Source: CAD feature listing. Evaluate the final solid. Frame: model axes, mm. Face numbers are marked on the shaded views. A direction names the side the tool comes from. Coordinates: 2 decimals unless noted, no trailing zeros. Write each loop counter-clockwise with the first axis right and the second up, starting at its lowest first coordinate (ties: lowest second). Pieces come first, ordered by that corner, then holes. Notation, with made-up numbers: (-23, -4.75) - (-19, -4.75) arc R33 ccw to (-19, 31.25) - close; hole circle Ø1 at (40, 56.5). An arc over 180 degrees is marked (long way). One line per question, with ' | ' between items.
from build123d import *

# Parameters (mm, degrees)
SKETCH1_R               = 17.5
BOSS_EXTRUDE1_DEPTH     = 4
BOSS_EXTRUDE2_DEPTH     = 6
CUT_EXTRUDE1_DEPTH      = 26.465663156
CUT_EXTRUDE1_DEPTH_BACK = 26.465663156
SKETCH3_R               = 1.6
CUT_EXTRUDE2_DEPTH      = 1
CUT_EXTRUDE2_DEPTH_BACK = 23.716032156
CUT_EXTRUDE2_START      = -2.749631
SKETCH5_R               = 2.1
CHAMFER1_SIZE           = 0.5
SKETCH6_R               = 3
CUT_EXTRUDE3_DEPTH      = 2


with BuildPart() as part:
    # Sketch1 → Boss-Extrude1 (new body)
    with BuildSketch(Plane(origin=(0, 0, 0), x_dir=(1, 0, 0), z_dir=(0, 1, 0))):
        with Locations(Location((0, 0, 0), (0, 0, 270))):
            Circle(SKETCH1_R)
    extrude(amount=BOSS_EXTRUDE1_DEPTH)

    # Sketch2 → Boss-Extrude2 (add)
    with BuildSketch(Plane(origin=(0, 0, 0), x_dir=(1, 0, 0), z_dir=(0, 1, 0))):
        with BuildLine():
            Line((-2.87, 6.929148577), (2.87, 6.929148577))
            ThreePointArc((2.87, 6.929148577), (0, -7.5), (-2.87, 6.929148577))
        make_face()
    extrude(amount=-BOSS_EXTRUDE2_DEPTH)

    # Sketch3 → Cut-Extrude1 (cut, two sides: drawn at the far end of the back side and taken through both)
    with BuildSketch(Plane(origin=(0, 0, 0), x_dir=(1, 0, 0), z_dir=(0, 1, 0)).offset(-CUT_EXTRUDE1_DEPTH_BACK)):
        with Locations(Location((0, 12.5, 0), (0, 0, 270))):
            Circle(SKETCH3_R)
        with Locations(Location((12.5, 0, 0), (0, 0, 270))):
            Circle(SKETCH3_R)
        with Locations(Location((0, -12.5, 0), (0, 0, 270))):
            Circle(SKETCH3_R)
        with Locations(Location((-12.5, 0, 0), (0, 0, 270))):
            Circle(SKETCH3_R)
        with BuildLine():
            Line((-1.5875, 2.749630657), (1.5875, 2.749630657))
            ThreePointArc((1.5875, 2.749630657), (0, -3.175), (-1.5875, 2.749630657))
        make_face()
    extrude(amount=CUT_EXTRUDE1_DEPTH + CUT_EXTRUDE1_DEPTH_BACK, mode=Mode.SUBTRACT)

    # Sketch5 → Cut-Extrude2 (cut, two sides: drawn at the far end of the back side and taken through both)
    with BuildSketch(Plane.XY.offset(CUT_EXTRUDE2_START - CUT_EXTRUDE2_DEPTH_BACK)):
        with Locations(Location((0, -3, 0), (0, 0, 180))):
            Circle(SKETCH5_R)
    extrude(amount=CUT_EXTRUDE2_DEPTH + CUT_EXTRUDE2_DEPTH_BACK, mode=Mode.SUBTRACT)

    # Chamfer1
    chamfer1_edges = [part.edges().sort_by_distance(p)[0] for p in [
        (2.1, -3, -6.929148577),
    ]]
    chamfer(chamfer1_edges, length=CHAMFER1_SIZE)

    # Sketch6 → Cut-Extrude3 (cut)
    with BuildSketch(Plane(origin=(0, 0, 0), x_dir=(1, 0, 0), z_dir=(0, 1, 0))):
        with Locations(Location((0, 12.5, 0), (0, 0, 270))):
            Circle(SKETCH6_R)
        with Locations(Location((12.5, 0, 0), (0, 0, 270))):
            Circle(SKETCH6_R)
        with Locations(Location((0, -12.5, 0), (0, 0, 270))):
            Circle(SKETCH6_R)
        with Locations(Location((-12.5, 0, 0), (0, 0, 270))):
            Circle(SKETCH6_R)
    extrude(amount=CUT_EXTRUDE3_DEPTH, mode=Mode.SUBTRACT)


solid = part.part
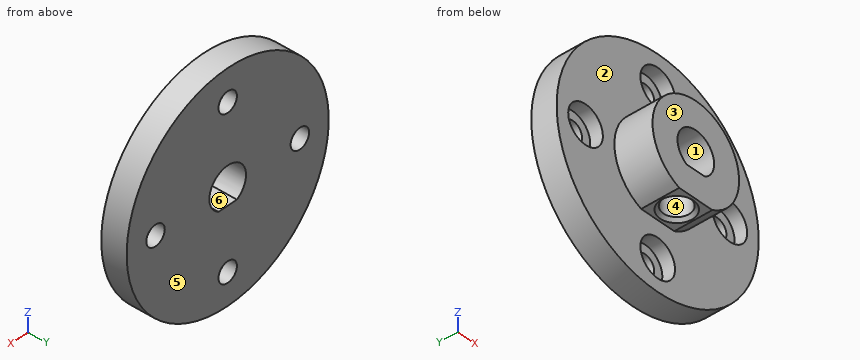
Item 1: Cut plane D-D on z = 12.5. Return loops of the section in (x, y), and give its area (3 significant figures).
Check sheet entries:
outline: (-12.25, 0) - (-3, 0) - (-3, 2) - (-1.6, 2) - (-1.6, 4) - (-12.25, 4) - close; (1.6, 2) - (3, 2) - (3, 0) - (12.25, 0) - (12.25, 4) - (1.6, 4) - close | area: 79.6 mm²
Item 2: Pin query (flat end, axial travel): pin 1 Ø0.5 at (x, y) = (-0.5, -5) entering from +Z; pin 2 Ø3 at (x, y) = (-8, 0) entering from +Z; pin 3 Ø4 at (x, z) = (0, 0) entering from -Y; pin 4 Ø5 at (y, z) = (-2, -5.5) entering from +X. Return the tip coordinate at first contact, or that it passes through.
Check sheet entries:
pin 1: z = 7.5 | pin 2: z = 16.25 | pin 3: through | pin 4: x = 17.04
Item 3: Cut plane B-B on z = 0. Return loops of the section in (x, y) (3 decimals), and give its area (3 significant figures).
Check sheet entries:
outline: (-17.5, 0) - (-15.5, 0) - (-15.5, 2) - (-14.1, 2) - (-14.1, 4) - (-17.5, 4) - close; (-10.9, 2) - (-9.5, 2) - (-9.5, 0) - (-7.5, 0) - (-7.5, -6) - (-3.175, -6) - (-3.175, 4) - (-10.9, 4) - close; (3.175, -6) - (7.5, -6) - (7.5, 0) - (9.5, 0) - (9.5, 2) - (10.9, 2) - (10.9, 4) - (3.175, 4) - close; (14.1, 2) - (15.5, 2) - (15.5, 0) - (17.5, 0) - (17.5, 4) - (14.1, 4) - close | area: 130 mm²
Item 4: Cut plane A-A on x = 0. State how many separate pieces and enclosed holes the cut face has, and give its area (3 significant figures).
Check sheet entries:
separate pieces: 5 | enclosed holes: 0 | area: 113 mm²
Item 5: Ray query, line 1 along Y through (x, z) = (-6.5, 5); line 2 along X through (y, z) = (-4.5, -3); line 3 along X through (y, z) = (-4.5, 1.5). Return the intervals inside material, ascending. Write a range as [from, to].
Check sheet entries:
line 1: [0, 4] | line 2: [-6.87, -1.47], [1.47, 6.87] | line 3: [-7.35, -2.8], [2.8, 7.35]
Item 6: Mould query, pull axis Y, two halves, no side actions, for the marked faces 3, 4, 5 and 6. Classes: pulls with the +Y half, pulls with the -Y half, needs draft (parallel to the pull), parting line crosses it, or undercut.
Check sheet entries:
face 3: pulls with the -Y half | face 4: undercut | face 5: pulls with the +Y half | face 6: needs draft
Item 7: Cut plane C-C on x = -12.5. Return loops of the section in (y, z).
Check sheet entries:
outline: (0, -12.25) - (4, -12.25) - (4, -1.6) - (2, -1.6) - (2, -3) - (0, -3) - close; (0, 3) - (2, 3) - (2, 1.6) - (4, 1.6) - (4, 12.25) - (0, 12.25) - close
Item 8: Access query for the marked faces 1 and 2. Directions: +Z, -Z, +X, -X, +Y, -Y. A direction counts if a zero-diameter tool reaches every point of the face in a straight line with its end or side. Return the directions, or none.
Check sheet entries:
face 1: +Y, -Y | face 2: -Y
